Autodesk Inventor part; units mm, degrees
ref_plane "YZ Plane" through (0, 0, 0) normal (1, 0, 0) x (0, 1, 0)
ref_plane "XZ Plane" through (0, 0, 0) normal (0, 1, 0) x (-1, 0, 0)
ref_plane "XY Plane" through (0, 0, 0) normal (0, 0, 1) x (1, 0, 0)
sketch "Sketch1" plane through (0, 0, 0) normal (0, 1, 0) x (-1, 0, 0)
  line L0 (0, 0) -> (-18.6, 0)
  line L1 (-18.6, 0) -> (-18.6, -41.3)
  line L2 (-18.6, -41.3) -> (0, -41.3)
  line L3 (0, -41.3) -> (0, 0)
  line L4 (-1.35, 0) -> (-1.35, -41.3)
  line L5 (0, -1.35) -> (-18.6, -1.35)
  line L6 (0, -39.95) -> (-18.6, -39.95)
  circle A0 centre (-2.85, -2.85) radius 1.5
  circle A1 centre (-2.85, -38.45) radius 1.5
  line L7 (-8.1, -22.5) -> (-14.6, -22.5)
  line L8 (-14.6, -22.5) -> (-14.6, -33)
  line L9 (-14.6, -33) -> (-8.1, -33)
  line L10 (-8.1, -33) -> (-8.1, -22.5)
  line L11 (-6.6, -1) -> (-17.6, -1)
  line L12 (-17.6, -1) -> (-17.6, -14)
  line L13 (-17.6, -14) -> (-6.6, -14)
  line L14 (-6.6, -14) -> (-6.6, -1)
  point P0 (-6.6, -1.35)
  point P1 (-17.6, -1.35)
  dimension "d0" = 18.6
  dimension "d1" = 41.3
  dimension "d2" = 1.35
  dimension "d3" = 1.35
  dimension "d4" = 1.35
  dimension "d5" = 3
  dimension "d6" = 3
  dimension "d7" = 6.5
  dimension "d8" = 10.5
  dimension "d11" = 8.1
  dimension "d12" = 8.3
  dimension "d13" = 11
  dimension "d14" = 13
  dimension "d16" = 1
  dimension "d17" = 1
extrude "Extrusion1" add sketch "Sketch1" against normal blind 0.8 contours L3 L5 L4 L0 | L4 L5 L14 L11 L12 L1 L0 | L3 L6 L4 L5 | L4 A0 L5 | L3 L2 L4 L6 | L5 L12 L13 L14 A0 L4 A1 L6 L1 | L6 A1 L4 | L4 L2 L1 L6 | L12 L11 L14 L5 | L5 L14 L13 L12 | L10 L9 L8 L7
extrude "Extrusion2" add sketch "Sketch1" along normal blind 4.5 contours L5 L14 L13 L12
extrude "Extrusion3" add sketch "Sketch1" along normal blind 4.5 contours L10 L9 L8 L7
chamfer "Chamfer1" distance 2 angle 45 2 edges at (8.1, 0, -27.75) (14.6, 0, -27.75)
properties part number "interface_board"
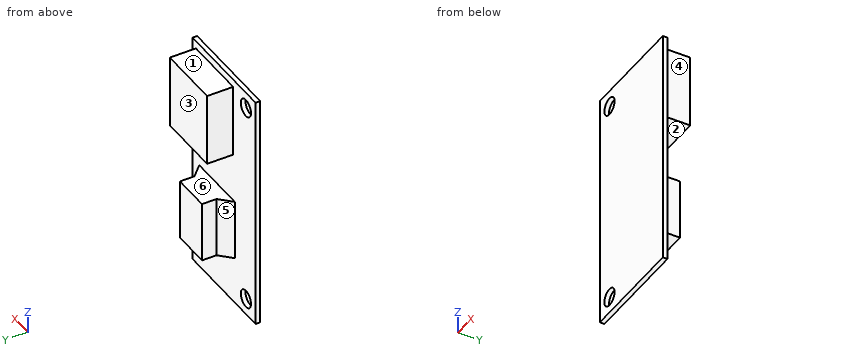
Here's how the part is built. I have some questions about the finished solid (model axes, mm). Face numbers are marked on the shaded views. A direction names the side the tool comes from. Round coordinates to 2 decimals unless told otherwise and drop trailing zeros. Order: outer loops, then holes, each group sorted by start corner. A loop starts at its lowest first (then second) coordinate and runs counter-clockwise, first axis right, second up. Notation, with made-up numbers: M -26,66 L 6,66 A14 cw 6,75 Z; hole C 9,-4.5 d5. An arc over 180 degrees is marked long. One line per question, with ' | ' between items.
1) I'm going to push flat-ended pins straight in: pin 1 Ø2 at (x, y) = (3.5, 2.5) entering from +Z; pin 2 Ø2 at (x, y) = (9.5, 3) entering from -Z; pin 3 Ø1.2 at (y, z) = (3, -25.5) entering from +X; pin 4 Ø1.3 at (x, y) = (9.5, 1.5) entering from +Z. Where does each tip first touch, or does it pass through?
Checked values:
pin 1: passes through | pin 2: stops at z = -33 | pin 3: stops at x = 14.6 | pin 4: stops at z = -1.35
2) Imagine slicing it at D-D, the plane x = 10. Write out the boundary of the cut face in (y, z), plus the area to 3 significant figures.
Checked values:
outline: M -0.8,-41.3 L 0,-41.3 L 0,-33 L 4.5,-33 L 4.5,-22.5 L 0,-22.5 L 0,-14 L 4.5,-14 L 4.5,-1.35 L 0,-1.35 L 0,0 L -0.8,0 Z | area: 137 mm²
3) Imagine slicing it at A-A, the plane x = 2.85. Write out the boundary of the cut face in (y, z), plus the area to 3 significant figures.
Checked values:
outline: M -0.8,-41.3 L 0,-41.3 L 0,-39.95 L -0.8,-39.95 Z; M -0.8,-36.95 L 0,-36.95 L 0,-4.35 L -0.8,-4.35 Z; M -0.8,-1.35 L 0,-1.35 L 0,0 L -0.8,0 Z | area: 28.2 mm²
4) We'd pull the mould along Z, two halves only. Please class the marked faces 1, 2 and 3: released by +Z, released by -Z, zero draft, split by the parting line, or undercut.
Checked values:
face 1: released by +Z | face 2: undercut | face 3: zero draft
5) Imagine slicing it at B-B, the plane y = 3.5. Write out the boundary of the cut face in (x, z), plus the area to 3 significant figures.
Checked values:
outline: M 6.6,-14 L 17.6,-14 L 17.6,-1.35 L 6.6,-1.35 Z; M 8.1,-33 L 14.6,-33 L 14.6,-22.5 L 8.1,-22.5 Z | area: 207 mm²
6) I need wall thicknesses on line 1 (Z direction, x = 2.85, y = -0.55); line 2 (X direction, y = -0.5, z = -2.85); line 3 (Z direction, x = 10, y = 1.35). Which ranges of each line are inside material? Lowest first, please.
Checked values:
line 1: z = -41.3 to -39.95, -36.95 to -4.35, -1.35 to 0 | line 2: x = 0 to 1.35, 4.35 to 18.6 | line 3: z = -33 to -22.5, -14 to -1.35
7) On a 3-axis mill with a long thin cutter (end or side, diameter ignored), from which of +Z, -Z, +X, -X, +Y, -Y can I reach the whole of each face in a straight line? I mean the marked faces 4, 5 and 6. Say none if no direction works.
Checked values:
face 4: +Z, -Z, +X, +Y | face 5: -Z, -X, +Y | face 6: +X, -X, +Y
8) Imagine slicing it at C-C, the plane z = -2.85. Write out the boundary of the cut face in (x, y), plus the area to 3 significant figures.
Checked values:
outline: M 0,-0.8 L 1.35,-0.8 L 1.35,0 L 0,0 Z; M 4.35,-0.8 L 18.6,-0.8 L 18.6,0 L 17.6,0 L 17.6,4.5 L 6.6,4.5 L 6.6,0 L 4.35,0 Z | area: 62.0 mm²
